Verification items for the finished model (mm, model axes). Face numbers are marked on the shaded views. A direction names the side the tool comes from. Round coordinates to 2 decimals unless told otherwise and drop trailing zeros. Write each loop counter-clockwise with the first axis right and the second up, starting at its lowest first coordinate (ties: lowest second). Pieces come first, ordered by that corner, then holes. Notation, with made-up numbers: (-12, 60) - (47, 60) arc R21 cw to (47, 98) - close; hole circle Ø4 at (-29, 8.25). An arc over 180 degrees is marked (long way). Answer as a JSON object with one key per item and string values.
```python
from build123d import *

# Parameters (mm, degrees)
SKETCH1_W           = 15
SKETCH1_H           = 18
BOSS_EXTRUDE1_DEPTH = 7
CUT_EXTRUDE1_DEPTH  = 16.2
SKETCH9_W           = 16
SKETCH9_H           = 6
BOSS_EXTRUDE2_DEPTH = 18
SKETCH13_W          = 16
SKETCH13_H          = 6
BOSS_EXTRUDE3_DEPTH = 18
SKETCH14_W          = 15
SKETCH14_H          = 3
CUT_EXTRUDE5_DEPTH  = 32.55
FILLET1_R           = 0.5


with BuildPart() as part:
    # Sketch1 → Boss-Extrude1 (new body)
    with BuildSketch(Plane(origin=(0, 0, 0), x_dir=(1, 0, 0), z_dir=(0, 1, 0))):
        Rectangle(SKETCH1_W, SKETCH1_H)
    extrude(amount=BOSS_EXTRUDE1_DEPTH)

    # Sketch2 → Cut-Extrude1 (cut)
    with BuildSketch(Plane.XY.offset(9)):
        Polygon((-2.25, 2.6), (-2.25, 0), (2.25, 0), (2.25, 2.6), (4.5, 2.6), (4.5, 4), (-4.5, 4), (-4.5, 2.6), align=None)
    extrude(amount=-CUT_EXTRUDE1_DEPTH, mode=Mode.SUBTRACT)

    # Sketch9 → Boss-Extrude2 (add)
    with BuildSketch(Plane.ZY.offset(7.5)):
        with Locations((0, 3)):
            Rectangle(SKETCH9_W, SKETCH9_H)
    extrude(amount=BOSS_EXTRUDE2_DEPTH)

    # Sketch13 → Boss-Extrude3 (add)
    with BuildSketch(Plane(origin=(7.5, 0, 0), x_dir=(0, 0, -1), z_dir=(1, 0, 0))):
        with Locations((0, 3)):
            Rectangle(SKETCH13_W, SKETCH13_H)
    extrude(amount=BOSS_EXTRUDE3_DEPTH)

    # Sketch14 → Cut-Extrude5 (cut)
    with BuildSketch(Plane.XY.offset(9)):
        with Locations((16.5, 4.5)):
            Rectangle(SKETCH14_W, SKETCH14_H)
        with Locations((-16.5, 4.5)):
            Rectangle(SKETCH14_W, SKETCH14_H)
    extrude(amount=-CUT_EXTRUDE5_DEPTH, mode=Mode.SUBTRACT)

    # Fillet1
    fillet1_edges = [part.edges().sort_by_distance(p)[0] for p in [
        (-7.5, 7, 0),
        (4.875, 0, 9),
        (0, 7, 9),
        (-2.25, 0, 0.9),
        (2.25, 0, 0.9),
        (-7.5, 0, 8.5),
        (-25.5, 6, 0),
        (7.5, 7, 0),
        (-4.875, 0, 9),
        (-7.5, 0, -8.5),
        (0, 0, -9),
        (7.5, 0, -8.5),
        (7.5, 0, 8.5),
        (25.5, 6, 0),
        (7.5, 3.5, 9),
        (-7.5, 3.5, 9),
        (-7.5, 3.5, -9),
        (9, 6, 0),
        (7.5, 3.5, -9),
        (0, 7, -9),
        (-9, 6, 0),
    ]]
    fillet(fillet1_edges, radius=FILLET1_R)


solid = part.part
```
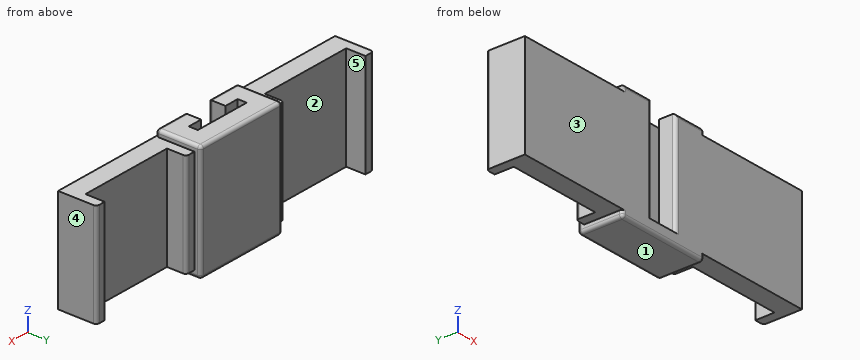
Q1. Set-up check for the marked faces 1 and 2: record each of +Z, -Z, +X, -X, +Y, -Y from which the full face is reachable in a straight line by a thin tool's end or side.
Geometry check:
{"face 1": "-Z, +X, -X, +Y, -Y", "face 2": "+Z, -Z, +Y"}
Q2. Section check A-A, the plane y = 4.75. Record the cut outline in (x, z).
Geometry check:
{"outline": "(-25.5, -8) - (-24, -8) - (-24, 8) - (-25.5, 8) - close; (-9, -8) - (-7.5, -8) - (-7.5, -8.5) arc R0.5 ccw to (-7, -9) - (7, -9) arc R0.5 ccw to (7.5, -8.5) - (7.5, -8) - (9, -8) - (9, 8) - (7.5, 8) - (7.5, 8.5) arc R0.5 ccw to (7, 9) - (-7, 9) arc R0.5 ccw to (-7.5, 8.5) - (-7.5, 8) - (-9, 8) - close; (24, -8) - (25.5, -8) - (25.5, 8) - (24, 8) - close"}
Q3. Section check C-C, the plane x = 0. Record the cut outline in (y, z).
Geometry check:
{"outline": "(0, -8.5) arc R0.5 ccw to (0.5, -9) - (6.5, -9) arc R0.5 ccw to (7, -8.5) - (7, 8.5) arc R0.5 ccw to (6.5, 9) - (4, 9) - (4, -7.2) - (0, -7.2) - close"}
Q4. Material ranges on line 1 along X through (y, z) = (3.5, 4); line 2 along X through (y, z) = (4.75, -5.5); line 3 along X through (y, z) = (2, -0.25), recorded low to high. Write a range as [from, to].
Geometry check:
{"line 1": "x = [-25.5, -24], [-9, -4.5], [4.5, 9], [24, 25.5]", "line 2": "x = [-25.5, -24], [-9, 9], [24, 25.5]", "line 3": "x = [-25.5, -2.25], [2.25, 25.5]"}
Q5. Release check for a two-part mould opening along X. For the marked faces 3, 4 and 5 record: released by +X, released by -X, zero draft, split by the parting line, or undercut.
Geometry check:
{"face 3": "zero draft", "face 4": "released by +X", "face 5": "undercut"}
Q6. Gauge pin test, flat ends, axial feed: P1, Ø1.5, axis at x = 9, y = 2.5, coming from the -Z side; P2, Ø1.1, axis at x = -24.5, z = 2, coming from the +Y side; P3, Ø1.2, axis at x = 2, y = 2.5, coming from the +Z side; P4, Ø4.5, axis at x = 20, z = -3.5, coming from the +Y side. Record the tip position at first contact, or that the pin passes through.
Geometry check:
{"P1": "stops at z = -8", "P2": "stops at y = 6", "P3": "stops at z = 9", "P4": "stops at y = 3"}
Q7. Section check D-D, the plane y = 1.75. Record the cut outline in (x, z).
Geometry check:
{"outline": "(-25.5, -8) - (-7.5, -8) - (-7.5, -8.5) arc R0.5 ccw to (-7, -9) - (7, -9) arc R0.5 ccw to (7.5, -8.5) - (7.5, -8) - (25.5, -8) - (25.5, 8) - (7.5, 8) - (7.5, 8.5) arc R0.5 ccw to (7, 9) - (2.25, 9) - (2.25, -7.2) - (-2.25, -7.2) - (-2.25, 9) - (-7, 9) arc R0.5 ccw to (-7.5, 8.5) - (-7.5, 8) - (-25.5, 8) - close"}
